For this review, take the finished solid that the model builds, in its own axes (mm). A direction names the side the tool comes from. Round coordinates to 2 decimals unless told otherwise and drop trailing zeros. Write each loop counter-clockwise with the first axis right and the second up, starting at its lowest first coordinate (ties: lowest second). Pieces come first, ordered by that corner, then holes. Notation, with made-up numbers: (7.25, -4) -> (46.25, -4) arc R19 cw to (46.25, 6) -> close; hole circle Ø4 at (16.5, -33.5). An arc over 180 degrees is marked (long way). Answer as CSV lines item,"result". Start each with the question number.
Item 1: Take a section at B-B on x = -7. Give the boundary of the cut face in (y, z), then the cut area to 3 significant figures.
Item 2: Take a section at A-A on z = 0. Give the boundary of the cut face in (x, y).
Item 3: Mouldability with a two-part tool opening along Z and no side actions: class faces 5 (the flat face through (0, -25, 0)), 6 (the flat face through (0, 0, -25)), 7 (the flat face through (-15, 12, 12)) as +Z half, -Z half, draft (parallel to the pull), parting line (faces both ways), or undercut.
Item 4: Take a section at D-D on y = 17. Give the boundary of the cut face in (x, z), then the cut area to 3 significant figures.
Item 5: For pin 1 Ø1.9 at (x, y) = (-2, -26) entering from +Z; pin 2 Ø2 at (y, z) = (-1, -12.5) entering from -X; pin 3 Ø1.9 at (x, z) = (-3.5, -27.5) entering from +Y; pin 4 Ø2 at (x, z) = (2, -11.5) entering from +Y, all flat-tipped, find the tip position at first contact; note any pin that passes through.
Item 6: Wall thickness on probe 1 along Z at (x, y) = (3.5, 0); probe 2 along Y at (x, z) = (-9, 0): over which ranges is each line inside the solid? List them lowest first. Write a range as from..to.
Item 7: Machinability: for faces 1 (the flat face through (0, -27, 2.5)), 2 (the flat face through (0, 2.5, -27)), 3 (the flat face through (0, -2.5, 27)), 4 (the flat face through (0, 27, -2.5)), which of the approach directions +Z, -Z, +X, -X, +Y, -Y give a long, thin tool a straight path to every point of the face, cutting with its end or side? Answer none if there is none.
Solid Edge part; units mm, degrees
sketch "Sketch1" plane through (0, 0, 0) normal (0, -1, 0) x (1, 0, 0)
  line L0 (-15, 15) -> (15, 15)
  line L1 (15, 15) -> (15, 29)
  line L2 (15, 29) -> (-15, 29)
  line L3 (-15, 29) -> (-15, 15)
  dimension "D1" = 15
revolve "RevolvedProtrusion1" add sketch "Sketch1" angle 360 about axis through (-60, 0, 0) along (1, 0, 0)
hole "Hole_1" at (15, 0, 0) direction (-1, 0, 0) diameter 42.587 depth 15 thread major 48 thread length 2
sketch "Sketch2" plane through (-15, 0, 0) normal (-1, 0, 0) x (0, -1, 0)
  line L0 (-2.5, 30) -> (2.5, 30)
  line L1 (2.5, 30) -> (2.5, 25)
  line L2 (2.5, 25) -> (-2.5, 25)
  line L3 (-2.5, 25) -> (-2.5, 30)
  dimension "D1" = 2.5
  dimension "D2" = 2.5
extrude "ExtrudedCutout_1" cut sketch "Sketch2" against normal blind 85.8062
pattern_circular "Pattern1" count 4 over 360 about axis through (-15, 0, 0) along (1, 0, 0) of "ExtrudedCutout_1"
Output values:
1,outline,"(-28.89, -2.5) arc R29 ccw to (-2.5, -28.89) -> (-2.5, -25) -> (2.5, -25) -> (2.5, -28.89) arc R29 ccw to (28.89, -2.5) -> (25, -2.5) -> (25, 2.5) -> (28.89, 2.5) arc R29 ccw to (2.5, 28.89) -> (2.5, 25) -> (-2.5, 25) -> (-2.5, 28.89) arc R29 ccw to (-28.89, 2.5) -> (-25, 2.5) -> (-25, -2.5) -> close; hole circle Ø30 at (0, 0)"
1,area,"1,860 mm^2"
2,outline,"(-15, -25) -> (15, -25) -> (15, -21.29) -> (0, -21.29) -> (0, -15) -> (-15, -15) -> close; (-15, 15) -> (0, 15) -> (0, 21.29) -> (15, 21.29) -> (15, 25) -> (-15, 25) -> close"
3,face 5,"undercut"
3,face 6,"-Z half"
3,face 7,"draft"
4,outline,"(-15, -23.49) -> (15, -23.49) -> (15, -12.82) -> (0, -12.82) -> (0, 12.82) -> (15, 12.82) -> (15, 23.49) -> (-15, 23.49) -> close"
4,area,"1,030 mm^2"
5,pin 1,"stops at z = 14.61"
5,pin 2,"passes through"
5,pin 3,"stops at y = 11.67"
5,pin 4,"stops at y = 27.03"
6,probe 1,"z = -25..-21.29, 21.29..25"
6,probe 2,"y = -25..-15, 15..25"
7,face 1,"+X, -X, -Y"
7,face 2,"-Z, +X, -X"
7,face 3,"+Z, +X, -X"
7,face 4,"+X, -X, +Y"
